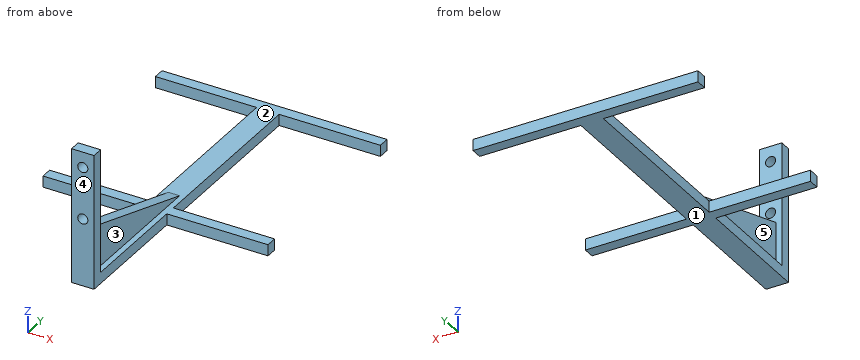
from build123d import *

# Parameters (mm, degrees)
SKETCH1_W               = 10
SKETCH1_H               = 60
BOSS_EXTRUDE1_DEPTH     = 5
SKETCH2_W               = 10
SKETCH2_H               = 5
BOSS_EXTRUDE2_DEPTH     = 140
RIB1_REACH              = 150.155
SKETCH3_WALL_W          = 365.362866258
SKETCH3_WALL_H          = 5
SKETCH4_W               = 100
SKETCH4_H               = 5
BOSS_EXTRUDE3_DEPTH     = 5
CUT_EXTRUDE1_DEPTH      = 152.657508881
CUT_EXTRUDE1_DEPTH_BACK = 152.657508881
SKETCH6_R               = 2.25


with BuildPart() as part:
    # Sketch1 → Boss-Extrude1 (new body)
    with BuildSketch(Plane(origin=(0, 0, 0), x_dir=(1, 0, 0), z_dir=(0, 1, 0))):
        Rectangle(SKETCH1_W, SKETCH1_H)
    extrude(amount=BOSS_EXTRUDE1_DEPTH)

    # Sketch2 → Boss-Extrude2 (add)
    with BuildSketch(Plane(origin=(0, 5, 0), x_dir=(1, 0, 0), z_dir=(0, 1, 0))):
        with Locations((0, 27.5)):
            Rectangle(SKETCH2_W, SKETCH2_H)
    extrude(amount=BOSS_EXTRUDE2_DEPTH)

    # Sketch3 wall → Rib1 (add, up to next)
    with BuildSketch(Plane(origin=(0, 37, -15), x_dir=(0, 0.954479978035, -0.298274993136), z_dir=(0, 0.298274993136, 0.954479978035)), mode=Mode.PRIVATE) as rib1_sk1:
        Rectangle(SKETCH3_WALL_W, SKETCH3_WALL_H)
    rib1_tool1 = extrude(rib1_sk1.sketch, amount=-RIB1_REACH, mode=Mode.PRIVATE) - part.part
    add(rib1_tool1.solids().sort_by_distance((0, 37, -15))[0])

    # Sketch4 → Boss-Extrude3 (add)
    with BuildSketch(Plane.XY.offset(-25)):
        with Locations((0, 142.5)):
            Rectangle(SKETCH4_W, SKETCH4_H)
        with Locations((0, 57.5)):
            Rectangle(SKETCH4_W, SKETCH4_H)
    extrude(amount=-BOSS_EXTRUDE3_DEPTH)

    # Sketch6 → Cut-Extrude1 (cut, two sides: drawn at the far end of the back side and taken through both)
    with BuildSketch(Plane(origin=(0, 5, 0), x_dir=(1, 0, 0), z_dir=(0, 1, 0)).offset(-CUT_EXTRUDE1_DEPTH_BACK)):
        with Locations(Location((0, 0, 0), (0, 0, 270))):
            Circle(SKETCH6_R)
        with Locations(Location((0, -23.103193392, 0), (0, 0, 270))):
            Circle(SKETCH6_R)
    extrude(amount=CUT_EXTRUDE1_DEPTH + CUT_EXTRUDE1_DEPTH_BACK, mode=Mode.SUBTRACT)


solid = part.part
Build history of the part. All positions in model axes, mm. Face numbers are marked on the shaded views. A direction names the side the tool comes from. Round coordinates to 2 decimals unless told otherwise and drop trailing zeros. Write each loop counter-clockwise with the first axis right and the second up, starting at its lowest first coordinate (ties: lowest second). Pieces come first, ordered by that corner, then holes. Notation, with made-up numbers: (64.5, 69) - (100.5, 69) arc R13 cw to (100.5, 75) - close; hole circle Ø4 at (32, 64). An arc over 180 degrees is marked (long way). Use CSV: the item, a comma, the result in double quotes.
(1) Band-saw the part on A-A (z = 0). Write the cut outline in (x, y), plus the area to 3 significant figures.
Response:
outline,"(-5, 0) - (-2.25, 0) - (-2.25, 5) - (-5, 5) - close; (2.25, 0) - (5, 0) - (5, 5) - (2.25, 5) - close"
area,"27.5 mm²"
(2) Wall check: line 1 (Z direction, x = 0, y = 2); line 2 (X direction, y = 2, z = 0); line 3 (Y direction, x = 1, z = 17.5). Give the ranges that are in metal, low to high.
Response:
line 1,"-30 to -2.25, 2.25 to 20.85, 25.35 to 30"
line 2,"-5 to -2.25, 2.25 to 5"
line 3,"0 to 5"
(3) Band-saw the part on D-D (y = 36). Write the cut outline in (x, z), plus the area to 3 significant figures.
Response:
outline,"(-5, -30) - (5, -30) - (5, -25) - (2.5, -25) - (2.5, -14.69) - (-2.5, -14.69) - (-2.5, -25) - (-5, -25) - close"
area,"102 mm²"
(4) 3-axis set-ups, long thin cutter, end or side, ignore diameter. For the marked faces 1, 2, 3, 4 and 5: which of +Z, -Z, +X, -X, +Y, -Y reach the whole face in a straight line?
Response:
face 1,"-Z, +X, -X, +Y, -Y"
face 2,"+Z, +Y"
face 3,"+Z, +X, +Y"
face 4,"+Z, -Z, +X, -X, -Y"
face 5,"+Z, -X, +Y"
(5) Band-saw the part on C-C (x = 20). Write the cut outline in (y, z), plus the area to 3 significant figures.
Response:
outline,"(55, -30) - (60, -30) - (60, -25) - (55, -25) - close; (140, -30) - (145, -30) - (145, -25) - (140, -25) - close"
area,"50.0 mm²"
(6) Pin check, flat tips, straight feed: P1, Ø1.5, axis at x = -29, z = -27.5, coming from the -Y side; P2, Ø6, axis at y = 48.5, z = -13, coming from the +X side (1 decimal); P3, Ø6, axis at y = 27, z = -12.5, coming from the -X side; P4, Ø5.5, axis at y = 111.5, z = -28, coming from the +X side. Stop position of each tip, or through.
Response:
P1,"y = 55"
P2,"through"
P3,"x = -2.5"
P4,"x = 5"
(7) Band-saw the part on B-B (x = 0). Write the cut outline in (y, z).
Response:
outline,"(0, -30) - (145, -30) - (145, -25) - (69, -25) - (5, -5) - (5, -2.25) - (0, -2.25) - close; (0, 2.25) - (5, 2.25) - (5, 20.85) - (0, 20.85) - close; (0, 25.35) - (5, 25.35) - (5, 30) - (0, 30) - close"
